Geometry: final body of the model. Coordinates: model frame, mm. A direction names the side the tool comes from. Coordinates: 2 decimals unless noted, no trailing zeros. Write each loop counter-clockwise with the first axis right and the second up, starting at its lowest first coordinate (ties: lowest second). Pieces come first, ordered by that corner, then holes.
from build123d import *

# Parameters (mm, degrees)
CROQUIS1_W              = 60
CROQUIS1_H              = 90
BASE_DEPTH              = 3.5
BASE_DEPTH_BACK         = 3.5
AGUJERO_SERVO_REACH     = 9
CROQUIS2_R              = 1
CROQUIS2_W              = 24.5
CROQUIS2_H              = 14.5
CROQUIS3_W              = 60
CROQUIS3_H              = 80
PARED_DEPTH             = 3.5
PARED_DEPTH_BACK        = 3.5
REDONDEO2_R             = 2
CROQUIS4_R              = 10
RECORTENUEVOSERVO_DEPTH = 2.5


with BuildPart() as part:
    # Croquis1 → Base (new body, two sides)
    with BuildSketch(Plane(origin=(0, 0, 0), x_dir=(1, 0, 0), z_dir=(0, 1, 0))) as base_sk:
        Rectangle(CROQUIS1_W, CROQUIS1_H)
    extrude(amount=BASE_DEPTH)
    extrude(base_sk.sketch, amount=-BASE_DEPTH_BACK)

    # Croquis2 → Agujero Servo (cut, up to next)
    with BuildSketch(Plane(origin=(0, 3.5, 0), x_dir=(1, 0, 0), z_dir=(0, 1, 0)), mode=Mode.PRIVATE) as agujero_servo_sk1:
        with Locations((-14, 25)):
            Circle(CROQUIS2_R)
    agujero_servo_tool1 = extrude(agujero_servo_sk1.sketch, amount=-AGUJERO_SERVO_REACH, mode=Mode.PRIVATE) & part.part
    add(agujero_servo_tool1.solids().sort_by_distance((-14, 3.5, -25))[0], mode=Mode.SUBTRACT)
    # Croquis2 → Agujero Servo (cut, up to next)
    with BuildSketch(Plane(origin=(0, 3.5, 0), x_dir=(1, 0, 0), z_dir=(0, 1, 0)), mode=Mode.PRIVATE) as agujero_servo_sk2:
        with Locations((14, 25)):
            Circle(CROQUIS2_R)
    agujero_servo_tool2 = extrude(agujero_servo_sk2.sketch, amount=-AGUJERO_SERVO_REACH, mode=Mode.PRIVATE) & part.part
    add(agujero_servo_tool2.solids().sort_by_distance((14, 3.5, -25))[0], mode=Mode.SUBTRACT)
    # Croquis2 → Agujero Servo (cut, up to next)
    with BuildSketch(Plane(origin=(0, 3.5, 0), x_dir=(1, 0, 0), z_dir=(0, 1, 0)), mode=Mode.PRIVATE) as agujero_servo_sk3:
        with Locations((0, 25)):
            Rectangle(CROQUIS2_W, CROQUIS2_H)
    agujero_servo_tool3 = extrude(agujero_servo_sk3.sketch, amount=-AGUJERO_SERVO_REACH, mode=Mode.PRIVATE) & part.part
    add(agujero_servo_tool3.solids().sort_by_distance((0, 3.5, -25))[0], mode=Mode.SUBTRACT)

    # Croquis3 → Pared (add, two sides)
    with BuildSketch(Plane.XY.offset(45)) as pared_sk:
        with Locations((0, 36.5)):
            Rectangle(CROQUIS3_W, CROQUIS3_H)
    extrude(amount=PARED_DEPTH)
    extrude(pared_sk.sketch, amount=-PARED_DEPTH_BACK)

    # Redondeo2
    redondeo2_edges = [part.edges().sort_by_distance(p)[0] for p in [
        (-30, -3.5, 1.75),
        (0, 3.5, -45),
        (-30, 3.5, -1.75),
        (30, -3.5, 1.75),
        (30, 3.5, -1.75),
        (-30, 40, 41.5),
        (0, 76.5, 41.5),
        (30, 40, 41.5),
        (-30, 36.5, 48.5),
        (0, -3.5, 48.5),
        (30, 36.5, 48.5),
        (0, 76.5, 48.5),
        (0, -3.5, -45),
    ]]
    fillet(redondeo2_edges, radius=REDONDEO2_R)

    # Croquis4 → RecorteNuevoServo (cut)
    with BuildSketch(Plane.XY.offset(48.5)):
        with Locations((0, 46.5)):
            Circle(CROQUIS4_R)
    extrude(amount=-RECORTENUEVOSERVO_DEPTH, mode=Mode.SUBTRACT)


solid = part.part
Item 1: Material intervals for probe 1 along X at (y, z) = (1, -25); probe 2 along Z at (x, y) = (14, 0.5); probe 3 along X at (y, z) = (-2, -25), sorted ascending.
Derived:
probe 1: x = -30 to -15, -13 to -12.25, 12.25 to 13, 15 to 30
probe 2: z = -45 to -26, -24 to 48.5
probe 3: x = -29.94 to -15, -13 to -12.25, 12.25 to 13, 15 to 29.94
Item 2: Pin query (flat end, axial travel): pin 1 (6 mm diameter, centred on y = 7, z = 33, fed in from +X); pin 2 (1.5 mm diameter, centred on x = -9, y = 68.5, fed in from -Z). Return the tip coordinate at first contact, or that it passes through.
Derived:
pin 1: passes through
pin 2: stops at z = 41.5
Item 3: Section A-A, the plane x = 0. Output: boundary loops of the cut face in (y, z).
Derived:
outline: (-3.5, -43) arc R2 ccw to (-1.5, -45) - (1.5, -45) arc R2 ccw to (3.5, -43) - (3.5, -32.25) - (-3.5, -32.25) - close; (-3.5, -17.75) - (3.5, -17.75) - (3.5, 41.5) - (74.5, 41.5) arc R2 ccw to (76.5, 43.5) - (76.5, 46.5) arc R2 ccw to (74.5, 48.5) - (56.5, 48.5) - (56.5, 46) - (36.5, 46) - (36.5, 48.5) - (-1.5, 48.5) arc R2 ccw to (-3.5, 46.5) - close
Item 4: Set-up query: faces 1 (the flat face through (0, 39, 41.5)), 2 (the flat face through (30, 0, 21)), 3 (the cylindrical face through (-2.17, 36.74, 47.27)), 4 (the flat face through (0, 0, -17.75)). Return all of +Z, -Z, +X, -X, +Y, -Y with unobstructed straight access to the full face (end or side cutting, diameter ignored); none if empty.
Derived:
face 1: -Z, +X, -X, +Y
face 2: +Z, -Z, +X, +Y, -Y
face 3: +Z
face 4: +Y, -Y
Item 5: Section D-D, the plane z = 7. Output: boundary loops of the cut face in (x, y), plus the area to 3 significant figures.
Derived:
outline: (-30, -1.5) arc R2 ccw to (-28, -3.5) - (28, -3.5) arc R2 ccw to (30, -1.5) - (30, 1.5) arc R2 ccw to (28, 3.5) - (-28, 3.5) arc R2 ccw to (-30, 1.5) - close
area: 417 mm2
Item 6: Pull-direction query (Y, two-part tool) for faces 5 (the flat face through (0, 47, 46)), 6 (the flat face through (0, 3.5, -1)), 7 (the flat face through (12.25, 0, -25)); classes: released by +Y, released by -Y, zero draft, split by the parting line, or undercut.
Derived:
face 5: undercut
face 6: released by +Y
face 7: zero draft
Item 7: Section C-C, the plane y = 46.5. Output: boundary loops of the cut face in (x, z), plus the area to 3 significant figures.
Derived:
outline: (-30, 43.5) arc R2 ccw to (-28, 41.5) - (28, 41.5) arc R2 ccw to (30, 43.5) - (30, 46.5) arc R2 ccw to (28, 48.5) - (10, 48.5) - (10, 46) - (-10, 46) - (-10, 48.5) - (-28, 48.5) arc R2 ccw to (-30, 46.5) - close
area: 367 mm2
Item 8: Section B-B, the plane x = 17. Output: boundary loops of the cut face in (y, z), plus the area to 3 significant figures.
Derived:
outline: (-3.5, -43) arc R2 ccw to (-1.5, -45) - (1.5, -45) arc R2 ccw to (3.5, -43) - (3.5, 41.5) - (74.5, 41.5) arc R2 ccw to (76.5, 43.5) - (76.5, 46.5) arc R2 ccw to (74.5, 48.5) - (-1.5, 48.5) arc R2 ccw to (-3.5, 46.5) - close
area: 1,160 mm2
